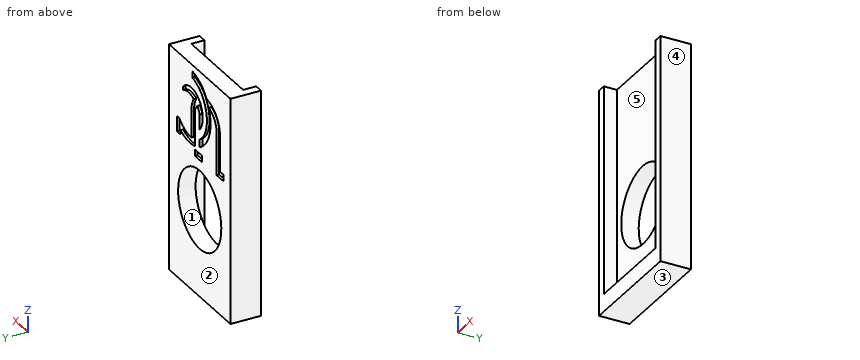
from build123d import *

# Parameters (mm, degrees)
SKETCH1_W           = 12.8
SKETCH1_H           = 25.9
SKETCH1_W_2         = 10.8
SKETCH1_H_2         = 21.9
BOSS_EXTRUDE1_DEPTH = 3.5
SKETCH3_W           = 10.8
SKETCH3_H           = 1.5
CUT_EXTRUDE1_DEPTH  = 15.863125512
SKETCH4_W           = 10.8
SKETCH4_H           = 21.9
SKETCH4_R           = 4.5
BOSS_EXTRUDE2_DEPTH = 2
SKETCH5_W           = 1.5
SKETCH5_H           = 0.75
CUT_EXTRUDE2_DEPTH  = 0.3


with BuildPart() as part:
    # Sketch1 → Boss-Extrude1 (new body)
    with BuildSketch(Plane(origin=(0, 0, 0), x_dir=(1, 0, 0), z_dir=(0, 1, 0))):
        Rectangle(SKETCH1_W, SKETCH1_H)
        Rectangle(SKETCH1_W_2, SKETCH1_H_2, mode=Mode.SUBTRACT)
    extrude(amount=BOSS_EXTRUDE1_DEPTH)

    # Sketch3 → Cut-Extrude1 (cut, through all)
    with BuildSketch(Plane.XY):
        with Locations((0, 0.75)):
            Rectangle(SKETCH3_W, SKETCH3_H)
    extrude(amount=CUT_EXTRUDE1_DEPTH, mode=Mode.SUBTRACT)

    # Sketch4 → Boss-Extrude2 (add)
    with BuildSketch(Plane(origin=(0, 3.5, 0), x_dir=(1, 0, 0), z_dir=(0, 1, 0))):
        Rectangle(SKETCH4_W, SKETCH4_H)
        with Locations(Location((0, 2.95, 0), (0, 0, 270))):
            Circle(SKETCH4_R, mode=Mode.SUBTRACT)
    extrude(amount=-BOSS_EXTRUDE2_DEPTH)

    # Sketch5 → Cut-Extrude2 (cut)
    with BuildSketch(Plane(origin=(0, 3.5, 0), x_dir=(1, 0, 0), z_dir=(0, 1, 0))):
        with BuildLine():
            Line((0, -6.25), (0, -8))
            ThreePointArc((0, -8), (0.216665991, -8.397222673), (0.5, -8.75))
            ThreePointArc((0.5, -8.75), (0.783334009, -8.397222673), (1, -8))
            Line((1, -8), (1, -3.86932209))
            ThreePointArc((1, -3.86932209), (2.535003662, -3.783808462), (4, -4.25))
            Line((4, -4.25), (4, -3.75))
            Line((4, -3.75), (4.75, -3.75))
            Line((4.75, -3.75), (4.75, -5.5))
            Line((4.75, -5.5), (4.25, -5.5))
            ThreePointArc((4.25, -5.5), (3.096291202, -4.759271996), (1.75, -4.5))
            Line((1.75, -4.5), (1.75, -7.5))
            ThreePointArc((1.75, -7.5), (1.622281323, -8.366025404), (1.25, -9.158312395))
            ThreePointArc((1.25, -9.158312395), (2.379117111, -9.416714281), (3.5, -9.124655157))
            Line((3.5, -9.124655157), (3.5, -9.5))
            ThreePointArc((3.5, -9.5), (0.408776976, -9.847754603), (-0.391896371, -6.841841224))
            ThreePointArc((-0.391896371, -6.841841224), (-0.215797248, -6.532777264), (0, -6.25))
        make_face()
        with BuildLine():
            Line((-4.25, -3.5), (-4.25, -7.5))
            ThreePointArc((-4.25, -7.5), (-3.437933175, -9.552546813), (-1.44136772, -10.493890178))
            ThreePointArc((-1.44136772, -10.493890178), (-0.151482732, -11.665190589), (1.5, -12.220485754))
            Line((1.5, -12.220485754), (1.5, -11.464101615))
            ThreePointArc((1.5, -11.464101615), (-1.405868052, -8.80626473), (0, -5.127718677))
            Line((0, -5.127718677), (0, -4.25))
            ThreePointArc((0, -4.25), (-2.016828361, -6.611623278), (-1.88878465, -9.714600228))
            ThreePointArc((-1.88878465, -9.714600228), (-2.929652546, -9.0783749), (-3.5, -8))
            Line((-3.5, -8), (-3.5, -2.75))
            Line((-3.5, -2.75), (-5, -2.75))
            Line((-5, -2.75), (-5, -3.5))
            Line((-5, -3.5), (-4.25, -3.5))
        make_face()
        with Locations((0.25, -3.125)):
            Rectangle(SKETCH5_W, SKETCH5_H)
    extrude(amount=-CUT_EXTRUDE2_DEPTH, mode=Mode.SUBTRACT)


solid = part.part
Source: CAD feature listing. Evaluate the final solid. Frame: model axes, mm. Face numbers are marked on the shaded views. A direction names the side the tool comes from. Round coordinates to 2 decimals unless told otherwise and drop trailing zeros. Order: outer loops, then holes, each group sorted by start corner. A loop starts at its lowest first (then second) coordinate and runs counter-clockwise, first axis right, second up. Notation, with made-up numbers: (-3.75, -11) -> (4.25, -11) arc R34 cw to (4.25, 28) -> close; hole circle Ø5 at (12.25, 46.25). An arc over 180 degrees is marked (long way). Answer as CSV lines item,"result".
Item 1: Section B-B, the plane x = 2.75. Return loops of the section in (y, z), plus the area to 3 significant figures.
A:
outline,"(0, -12.95) -> (3.5, -12.95) -> (3.5, -6.51) -> (1.5, -6.51) -> (1.5, -10.95) -> (0, -10.95) -> close; (1.5, 0.61) -> (3.5, 0.61) -> (3.5, 3.82) -> (3.2, 3.82) -> (3.2, 4.64) -> (3.5, 4.64) -> (3.5, 9.38) -> (3.2, 9.38) -> (3.2, 10.04) -> (3.5, 10.04) -> (3.5, 12.95) -> (1.5, 12.95) -> close"
area,"40.1 mm²"
Item 2: Pin query (flat end, axial travel): pin 1 Ø1.6 at (x, y) = (-2.5, 0.5) entering from +Z. Return the tip coordinate at first contact, or that it passes through.
A:
pin 1,"z = -10.95"
Item 3: Pull-direction query (Z, two-part tool) for the marked faces 1, 2 and 3; classes: pulls with the +Z half, pulls with the -Z half, needs draft (parallel to the pull), parting line crosses it, or undercut.
A:
face 1,"undercut"
face 2,"needs draft"
face 3,"pulls with the -Z half"
Item 4: Reachability of the marked faces 4 and 5 from +Z, -Z, +X, -X, +Y, -Y: full face, straight path, thin tool, end or side. Return the list, or none.
A:
face 4,"+Z, -Z, +X, +Y, -Y"
face 5,"+Z, -Y"
Item 5: Section D-D, the plane y = 0.35. Return loops of the section in (x, z), plus the area to 3 significant figures.
A:
outline,"(-6.4, -12.95) -> (6.4, -12.95) -> (6.4, 12.95) -> (5.4, 12.95) -> (5.4, -10.95) -> (-5.4, -10.95) -> (-5.4, 12.95) -> (-6.4, 12.95) -> close"
area,"73.4 mm²"
Item 6: Section C-C, the plane y = 2.8. Return loops of the section in (x, z), plus the area to 3 significant figures.
A:
outline,"(-6.4, -12.95) -> (6.4, -12.95) -> (6.4, 12.95) -> (-6.4, 12.95) -> close; hole circle Ø9 at (0, -2.95)"
area,"268 mm²"
Item 7: Section A-A, the plane z = -2.95. Return loops of the section in (x, y), plus the area to 3 significant figures.
A:
outline,"(-6.4, 0) -> (-5.4, 0) -> (-5.4, 1.5) -> (-4.5, 1.5) -> (-4.5, 3.5) -> (-6.4, 3.5) -> close; (4.5, 1.5) -> (5.4, 1.5) -> (5.4, 0) -> (6.4, 0) -> (6.4, 3.5) -> (4.5, 3.5) -> close"
area,"10.6 mm²"
Item 8: Line query: L1, parallel to X at y = 2.55, z = -2.95; L2, parallel to X at y = 1.05, z = 9.75; L3, parallel to Y at x = 2, z = -9. Output: solid intervals per line, ascending.
A:
L1,"-6.4 to -4.5, 4.5 to 6.4"
L2,"-6.4 to -5.4, 5.4 to 6.4"
L3,"1.5 to 3.5"
